from build123d import *

# Parameters (mm, degrees)
EXTRUDE_THIN1_DEPTH = 217.4875


with BuildPart() as part:
    # Sketch1 → Extrude-Thin1 (new body)
    with BuildSketch(Plane(origin=(0, 0, 0), x_dir=(0, 0, -1), z_dir=(1, 0, 0))):
        with BuildLine():
            ThreePointArc((0.614869388, 0.207178861), (0.324417726, 0.053186862), (0, 0))
            Line((0, 0), (-2.5146, 0))
            Line((-2.5146, 0), (-2.5146, 0.127))
            Line((-2.5146, 0.127), (0, 0.127))
            ThreePointArc((0, 0.127), (0.283865511, 0.173538504), (0.538010715, 0.308281503))
            Line((0.538010715, 0.308281503), (0.614869388, 0.207178861))
        make_face()
    extrude(amount=-EXTRUDE_THIN1_DEPTH)


solid = part.part
CAD build for the part. Positions are in the model's coordinates, mm. Round coordinates to 2 decimals unless told otherwise and drop trailing zeros. Write each loop counter-clockwise with the first axis right and the second up, starting at its lowest first coordinate (ties: lowest second). Pieces come first, ordered by that corner, then holes. Notation, with made-up numbers: M 23.25,34.25 L 47.25,34.25 A21 ccw 47.25,71.25 Z; hole C 45,16.25 d9. An arc over 180 degrees is marked long. Use a Markdown table: item, result. Add a question column.
1. Slice it at C-C on y = 0.05. Give the cut face in (x, z), then the cut area to 3 significant figures.
2. Slice it at A-A on x = -146.5. Give the cut face in (y, z).
3. Slice it at B-B on z = 0.75. Give the cut face in (x, y).
4. Flat gauge pin, fed straight in: P1, Ø1.5, axis at x = -103, z = 1.5, coming from the -Y side. Where does the tip first touch, or does it go through?
Reply:
| question | item | result |
|---|---|---|
| 1 | outline | M -217.49,-0.31 L 0,-0.31 L 0,2.51 L -217.49,2.51 Z |
| 1 | area | 615 mm^2 |
| 2 | outline | M 0,0 A1.02 ccw 0.21,-0.61 L 0.31,-0.54 A0.89 cw 0.13,0 L 0.13,2.51 L 0,2.51 Z |
| 3 | outline | M -217.49,0 L 0,0 L 0,0.13 L -217.49,0.13 Z |
| 4 | P1 | stops at y = 0 |
